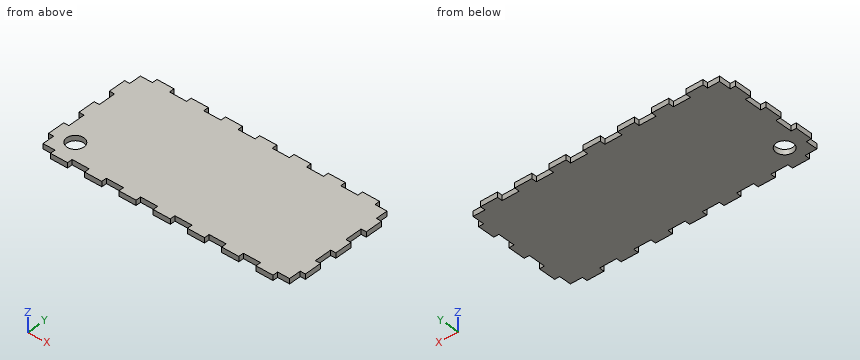
from build123d import *

# Parameters (mm, degrees)
SKETCH1_W               = 150
SKETCH1_H               = 70
BOSS_EXTRUDE1_DEPTH     = 3
SKETCH2_W               = 10
SKETCH2_H               = 3
CUT_EXTRUDE1_DEPTH      = 3
LPATTERN3_COUNT         = 8
LPATTERN3_PITCH         = 20
MIRROR1_COPY_1_SKETCH_W = 10
MIRROR1_COPY_1_SKETCH_H = 3
MIRROR1_COPY_1_DEPTH    = 3
MIRROR1_COPY_2_SKETCH_W = 10
MIRROR1_COPY_2_SKETCH_H = 3
MIRROR1_COPY_2_DEPTH    = 3
MIRROR1_COPY_3_SKETCH_W = 10
MIRROR1_COPY_3_SKETCH_H = 3
MIRROR1_COPY_3_DEPTH    = 3
MIRROR1_COPY_4_SKETCH_W = 10
MIRROR1_COPY_4_SKETCH_H = 3
MIRROR1_COPY_4_DEPTH    = 3
MIRROR1_COPY_5_SKETCH_W = 10
MIRROR1_COPY_5_SKETCH_H = 3
MIRROR1_COPY_5_DEPTH    = 3
MIRROR1_COPY_6_SKETCH_W = 10
MIRROR1_COPY_6_SKETCH_H = 3
MIRROR1_COPY_6_DEPTH    = 3
MIRROR1_COPY_7_SKETCH_W = 10
MIRROR1_COPY_7_SKETCH_H = 3
MIRROR1_COPY_7_DEPTH    = 3
SKETCH3_W               = 3
SKETCH3_H               = 10
CUT_EXTRUDE2_DEPTH      = 3
LPATTERN4_COUNT         = 4
LPATTERN4_PITCH         = 20
MIRROR2_COPY_1_SKETCH_W = 3
MIRROR2_COPY_1_SKETCH_H = 10
MIRROR2_COPY_1_DEPTH    = 3
MIRROR2_COPY_2_SKETCH_W = 3
MIRROR2_COPY_2_SKETCH_H = 10
MIRROR2_COPY_2_DEPTH    = 3
MIRROR2_COPY_3_SKETCH_W = 3
MIRROR2_COPY_3_SKETCH_H = 10
MIRROR2_COPY_3_DEPTH    = 3
SKETCH6_R               = 5
CUT_EXTRUDE3_DEPTH      = 3


with BuildPart() as part:
    # Sketch1 → Boss-Extrude1 (new body)
    with BuildSketch(Plane.XY):
        Rectangle(SKETCH1_W, SKETCH1_H)
    extrude(amount=BOSS_EXTRUDE1_DEPTH)

    # Sketch2 → Cut-Extrude1 (cut)
    with BuildSketch(Plane.XY.offset(3)):
        with Locations((-70, 33.5)):
            Rectangle(SKETCH2_W, SKETCH2_H)
    cut_extrude1 = extrude(amount=-CUT_EXTRUDE1_DEPTH, mode=Mode.SUBTRACT)

    # LPattern3: Cut-Extrude1 ×8
    with Locations(*[(i * LPATTERN3_PITCH, 0, 0) for i in range(1, LPATTERN3_COUNT)]):
        add(cut_extrude1, mode=Mode.SUBTRACT)

    # Mirror1: Cut-Extrude1 across plane
    add(cut_extrude1.mirror(Plane.ZX), mode=Mode.SUBTRACT)

    # Mirror1 copy 1 sketch → Mirror1 copy 1 (cut)
    with BuildSketch(Plane(origin=(20, 0, 3), x_dir=(1, 0, 0), z_dir=(0, 0, 1))):
        with Locations((-70, -33.5)):
            Rectangle(MIRROR1_COPY_1_SKETCH_W, MIRROR1_COPY_1_SKETCH_H)
    extrude(amount=-MIRROR1_COPY_1_DEPTH, mode=Mode.SUBTRACT)

    # Mirror1 copy 2 sketch → Mirror1 copy 2 (cut)
    with BuildSketch(Plane(origin=(40, 0, 3), x_dir=(1, 0, 0), z_dir=(0, 0, 1))):
        with Locations((-70, -33.5)):
            Rectangle(MIRROR1_COPY_2_SKETCH_W, MIRROR1_COPY_2_SKETCH_H)
    extrude(amount=-MIRROR1_COPY_2_DEPTH, mode=Mode.SUBTRACT)

    # Mirror1 copy 3 sketch → Mirror1 copy 3 (cut)
    with BuildSketch(Plane(origin=(60, 0, 3), x_dir=(1, 0, 0), z_dir=(0, 0, 1))):
        with Locations((-70, -33.5)):
            Rectangle(MIRROR1_COPY_3_SKETCH_W, MIRROR1_COPY_3_SKETCH_H)
    extrude(amount=-MIRROR1_COPY_3_DEPTH, mode=Mode.SUBTRACT)

    # Mirror1 copy 4 sketch → Mirror1 copy 4 (cut)
    with BuildSketch(Plane(origin=(80, 0, 3), x_dir=(1, 0, 0), z_dir=(0, 0, 1))):
        with Locations((-70, -33.5)):
            Rectangle(MIRROR1_COPY_4_SKETCH_W, MIRROR1_COPY_4_SKETCH_H)
    extrude(amount=-MIRROR1_COPY_4_DEPTH, mode=Mode.SUBTRACT)

    # Mirror1 copy 5 sketch → Mirror1 copy 5 (cut)
    with BuildSketch(Plane(origin=(100, 0, 3), x_dir=(1, 0, 0), z_dir=(0, 0, 1))):
        with Locations((-70, -33.5)):
            Rectangle(MIRROR1_COPY_5_SKETCH_W, MIRROR1_COPY_5_SKETCH_H)
    extrude(amount=-MIRROR1_COPY_5_DEPTH, mode=Mode.SUBTRACT)

    # Mirror1 copy 6 sketch → Mirror1 copy 6 (cut)
    with BuildSketch(Plane(origin=(120, 0, 3), x_dir=(1, 0, 0), z_dir=(0, 0, 1))):
        with Locations((-70, -33.5)):
            Rectangle(MIRROR1_COPY_6_SKETCH_W, MIRROR1_COPY_6_SKETCH_H)
    extrude(amount=-MIRROR1_COPY_6_DEPTH, mode=Mode.SUBTRACT)

    # Mirror1 copy 7 sketch → Mirror1 copy 7 (cut)
    with BuildSketch(Plane(origin=(140, 0, 3), x_dir=(1, 0, 0), z_dir=(0, 0, 1))):
        with Locations((-70, -33.5)):
            Rectangle(MIRROR1_COPY_7_SKETCH_W, MIRROR1_COPY_7_SKETCH_H)
    extrude(amount=-MIRROR1_COPY_7_DEPTH, mode=Mode.SUBTRACT)

    # Sketch3 → Cut-Extrude2 (cut)
    with BuildSketch(Plane.XY.offset(3)):
        with Locations((-73.5, 30)):
            Rectangle(SKETCH3_W, SKETCH3_H)
    cut_extrude2 = extrude(amount=-CUT_EXTRUDE2_DEPTH, mode=Mode.SUBTRACT)

    # LPattern4: Cut-Extrude2 ×4
    with Locations(*[(0, -i * LPATTERN4_PITCH, 0) for i in range(1, LPATTERN4_COUNT)]):
        add(cut_extrude2, mode=Mode.SUBTRACT)

    # Mirror2: Cut-Extrude2 across plane
    add(cut_extrude2.mirror(Plane(origin=(0, 0, 0), x_dir=(0, 0, 1), z_dir=(1, 0, 0))), mode=Mode.SUBTRACT)

    # Mirror2 copy 1 sketch → Mirror2 copy 1 (cut)
    with BuildSketch(Plane(origin=(0, -20, 3), x_dir=(-1, 0, 0), z_dir=(0, 0, 1))):
        with Locations((-73.5, -30)):
            Rectangle(MIRROR2_COPY_1_SKETCH_W, MIRROR2_COPY_1_SKETCH_H)
    extrude(amount=-MIRROR2_COPY_1_DEPTH, mode=Mode.SUBTRACT)

    # Mirror2 copy 2 sketch → Mirror2 copy 2 (cut)
    with BuildSketch(Plane(origin=(0, -40, 3), x_dir=(-1, 0, 0), z_dir=(0, 0, 1))):
        with Locations((-73.5, -30)):
            Rectangle(MIRROR2_COPY_2_SKETCH_W, MIRROR2_COPY_2_SKETCH_H)
    extrude(amount=-MIRROR2_COPY_2_DEPTH, mode=Mode.SUBTRACT)

    # Mirror2 copy 3 sketch → Mirror2 copy 3 (cut)
    with BuildSketch(Plane(origin=(0, -60, 3), x_dir=(-1, 0, 0), z_dir=(0, 0, 1))):
        with Locations((-73.5, -30)):
            Rectangle(MIRROR2_COPY_3_SKETCH_W, MIRROR2_COPY_3_SKETCH_H)
    extrude(amount=-MIRROR2_COPY_3_DEPTH, mode=Mode.SUBTRACT)

    # Sketch6 → Cut-Extrude3 (cut)
    with BuildSketch(Plane(origin=(0, 0, 0), x_dir=(-1, 0, 0), z_dir=(0, 0, -1))):
        with Locations((62, -22)):
            Circle(SKETCH6_R)
    extrude(amount=-CUT_EXTRUDE3_DEPTH, mode=Mode.SUBTRACT)


solid = part.part
Check sheet for the modelled part. Datum: model origin and axes. Units: mm. Give positions to 0.01 mm unless a question says otherwise; leave off trailing zeros. Order: outer loops, then holes, each group sorted by start corner. A loop starts at its lowest first (then second) coordinate and runs counter-clockwise, first axis right, second up. Notation, with made-up numbers: (71, 28.25) - (75, 28.25) arc R10 ccw to (75, 36.25) - close; hole circle Ø11 at (45, 5.25). An arc over 180 degrees is marked (long way). Answer as CSV lines item,"result".
1. Scan lines: probe 1 along Y at (x, z) = (-62, 2.35); probe 2 along X at (y, z) = (30.5, 1.9); probe 3 along X at (y, z) = (-20.5, 1.35). Record each from-to range of solid material in increasing order. Write a range as from..to.
Result sheet:
probe 1,"-35..-27, -17..35"
probe 2,"-72..72"
probe 3,"-75..-66.77, -57.23..75"
2. Section check B-B (y = -22). Record the boundary of the cut face in (x, z), then the cut area to 3 significant figures.
Result sheet:
outline,"(-75, 0) - (-67, 0) - (-67, 3) - (-75, 3) - close; (-57, 0) - (75, 0) - (75, 3) - (-57, 3) - close"
area,"420 mm²"
3. Section check A-A (x = -62). Record the boundary of the cut face in (y, z).
Result sheet:
outline,"(-35, 0) - (-27, 0) - (-27, 3) - (-35, 3) - close; (-17, 0) - (35, 0) - (35, 3) - (-17, 3) - close"
4. Go/stop test with flat-tipped pins: P1, Ø0.9, axis at y = 28, z = 1, coming from the +X side; P2, Ø0.9, axis at y = -33.5, z = 1, coming from the -X side; P3, Ø1.5, axis at y = 33.5, z = 1, coming from the +X side. Record where each tip stops, or that it passes through.
Result sheet:
P1,"x = 72"
P2,"x = -65"
P3,"x = 65"
5. Section check C-C (x = 13.5). Record the boundary of the cut face in (y, z).
Result sheet:
outline,"(-32, 0) - (32, 0) - (32, 3) - (-32, 3) - close"
6. Section check D-D (y = 9.5). Record the boundary of the cut face in (x, z).
Result sheet:
outline,"(-72, 0) - (72, 0) - (72, 3) - (-72, 3) - close"
